Can you work these out from the model? Positions are in its coordinate system, mm. Face numbers are marked on the shaded views. A direction names the side the tool comes from. Give positions to 0.01 mm unless a question says otherwise; leave off trailing zeros. Write each loop counter-clockwise with the first axis right and the second up, starting at its lowest first coordinate (ties: lowest second). Pieces come first, ordered by that corner, then holes.
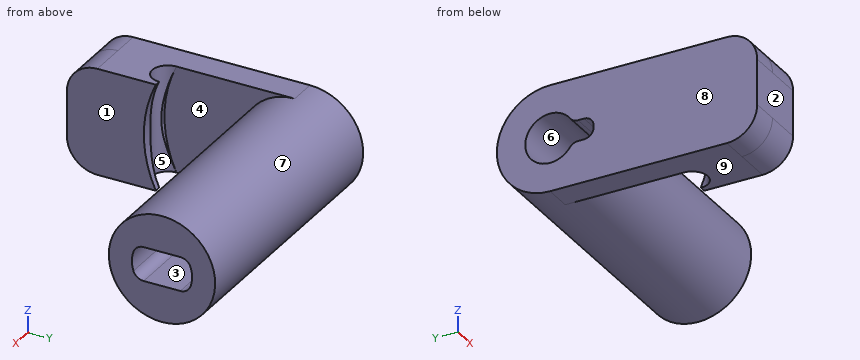
from build123d import *

# Parameters (mm, degrees)
SKETCH1_R           = 8.7376
BOSS_EXTRUDE1_DEPTH = 43.815
BOSS_EXTRUDE3_DEPTH = 4.516000112
FILLET2_R           = 5
BOSS_EXTRUDE4_START = 6.096
BOSS_EXTRUDE4_DEPTH = 6.096
CUT_EXTRUDE8_DEPTH  = 6.096
CUT_EXTRUDE10_DEPTH = 12.192
FILLET11_R          = 1.778
SKETCH25_R          = 2.5527
CUT_EXTRUDE14_DEPTH = 59.168600946
CUT_EXTRUDE15_DEPTH = 21.59
FILLET12_R          = 1.5875


with BuildPart() as part:
    # Sketch1 → Boss-Extrude1 (new body)
    with BuildSketch(Plane.YZ):
        with Locations(Location((0, 0, 0), (0, 0, 270))):
            Circle(SKETCH1_R)
    extrude(amount=BOSS_EXTRUDE1_DEPTH)

    # Sketch10 → Boss-Extrude3 (add)
    with BuildSketch(Plane(origin=(0, 0, 0), x_dir=(0, -1, 0), z_dir=(-1, 0, 0))):
        with BuildLine():
            Line((0, 8.7376), (34.036, 8.7376))
            Line((34.036, 8.7376), (34.036, -8.7376))
            Line((34.036, -8.7376), (0, -8.7376))
            ThreePointArc((0, -8.7376), (8.7376, 0), (0, 8.7376))
        make_face()
    extrude(amount=-BOSS_EXTRUDE3_DEPTH)

    # Fillet2
    fillet2_edges = [part.edges().sort_by_distance(p)[0] for p in [
        (2.258000056, -34.036, 8.7376),
        (2.258000056, -34.036, -8.7376),
    ]]
    fillet(fillet2_edges, radius=FILLET2_R)

    # Sketch15 → Boss-Extrude4 (add)
    with BuildSketch(Plane.YZ.offset(4.516000112).offset(BOSS_EXTRUDE4_START)):
        with BuildLine():
            Line((-18.796, 8.7376), (-29.036, 8.7376))
            ThreePointArc((-29.036, 8.7376), (-32.571533906, 7.273133906), (-34.036, 3.7376))
            Line((-34.036, 3.7376), (-34.036, -3.7376))
            ThreePointArc((-34.036, -3.7376), (-32.571533906, -7.273133906), (-29.036, -8.7376))
            Line((-29.036, -8.7376), (-18.796, -8.7376))
            Line((-18.796, -8.7376), (-18.796, 8.7376))
        make_face()
    extrude(amount=-BOSS_EXTRUDE4_DEPTH)

    # Sketch21 → Cut-Extrude8 (cut)
    with BuildSketch(Plane.YZ.offset(10.612000112)):
        with BuildLine():
            Line((-19.431, -8.7376), (-18.796, -8.7376))
            Line((-18.796, -8.7376), (-18.796, 8.7376))
            Line((-18.796, 8.7376), (-19.431, 8.7376))
            ThreePointArc((-19.431, 8.7376), (-21.405517007, 0), (-19.431, -8.7376))
        make_face()
    extrude(amount=-CUT_EXTRUDE8_DEPTH, mode=Mode.SUBTRACT)

    # Sketch22 → Cut-Extrude10 (cut)
    with BuildSketch(Plane.YZ.offset(43.815)):
        with BuildLine():
            Line((-4.089715516, -2.794), (4.089715516, -2.794))
            ThreePointArc((4.089715516, -2.794), (4.953, 0), (4.089715516, 2.794))
            Line((4.089715516, 2.794), (-4.089715516, 2.794))
            ThreePointArc((-4.089715516, 2.794), (-4.953, 0), (-4.089715516, -2.794))
        make_face()
    extrude(amount=-CUT_EXTRUDE10_DEPTH, mode=Mode.SUBTRACT)

    # Fillet11
    fillet11_edges = [part.edges().sort_by_distance(p)[0] for p in [
        (37.719, 4.089715516, 2.794),
        (37.719, 4.089715516, -2.794),
        (37.719, -4.089715516, -2.794),
        (37.719, -4.089715516, 2.794),
    ]]
    fillet(fillet11_edges, radius=FILLET11_R)

    # Sketch25 → Cut-Extrude14 (cut, through all)
    with BuildSketch(Plane(origin=(0, 0, -8.7376), x_dir=(1, 0, 0), z_dir=(0, 0, -1))):
        with Locations((7.068700112, 19.431)):
            Circle(SKETCH25_R)
    extrude(amount=-CUT_EXTRUDE14_DEPTH, mode=Mode.SUBTRACT)

    # Sketch26 → Cut-Extrude15 (cut)
    with BuildSketch(Plane(origin=(0, 0, 0), x_dir=(0, -1, 0), z_dir=(-1, 0, 0))):
        with BuildLine():
            Line((3.684641875, 1.7145), (7.177141875, 1.7145))
            Line((7.177141875, 1.7145), (7.177141875, -1.7145))
            Line((7.177141875, -1.7145), (3.684641875, -1.7145))
            ThreePointArc((3.684641875, -1.7145), (-4.064, 0), (3.684641875, 1.7145))
        make_face()
    extrude(amount=-CUT_EXTRUDE15_DEPTH, mode=Mode.SUBTRACT)

    # Fillet12
    fillet12_edges = [part.edges().sort_by_distance(p)[0] for p in [
        (10.795, -3.684641875, -1.7145),
        (10.795, -3.684641875, 1.7145),
        (10.795, -7.177141875, 1.7145),
        (10.795, -7.177141875, -1.7145),
    ]]
    fillet(fillet12_edges, radius=FILLET12_R)


solid = part.part
(1) Imagine slicing it at B-B, the plane z = -7.5. Write out the boundary of the cut face in (x, y) (3 decimals).
Returned:
outline: (0, -32.329) - (10.612, -32.329) - (10.612, -19.971) - (9.564, -19.971) arc R2.553 cw to (4.574, -19.971) - (4.516, -19.971) - (4.516, -4.483) - (43.815, -4.483) - (43.815, 4.483) - (0, 4.483) - close
(2) Will these pins go through, and if not, where does the flat tip stop? P1, Ø6, axis at x = 25.5, z = 3.5, coming from the -Y side; P2, Ø4.5, axis at y = -0.5, z = -1, coming from the +X side (3 decimals); P3, Ø6, axis at y = -18, z = 0.5, coming from the +X side; P4, Ø6, axis at y = -24.5, z = 0.5, coming from the +X side.
Returned:
P1: stops at y = -8.72
P2: stops at x = 43.815
P3: stops at x = 4.52
P4: stops at x = 10.61
(3) Imagine slicing it at D-D, the plane y = 2. Write out the boundary of the cut face in (x, z) (3 decimals), plus the area to 3 significant figures.
Returned:
outline: (0, -8.506) - (43.815, -8.506) - (43.815, -2.794) - (31.623, -2.794) - (31.623, 2.794) - (43.815, 2.794) - (43.815, 8.506) - (0, 8.506) - (0, 3.538) - (21.59, 3.538) - (21.59, -3.538) - (0, -3.538) - close
area: 524 mm2
(4) Imagine slicing it at C-C, the plane x = 35. Write out the boundary of the cut face in (y, z).
Returned:
outline: circle Ø17.48 at (0, 0); hole (-4.69, -1.58) arc R1.78 ccw to (-3.01, -2.79) - (3.01, -2.79) arc R1.78 ccw to (4.69, -1.58) arc R4.95 ccw to (4.69, 1.58) arc R1.78 ccw to (3.01, 2.79) - (-3.01, 2.79) arc R1.78 ccw to (-4.69, 1.58) arc R4.95 ccw to start
(5) For the marked faces 5, 6, 7, 8 and 9, which set-ups out of +Z, -Z, +X, -X, +Y, -Y let a thin tool reach every point of the face, with its end or its side?
Returned:
face 5: +Z, -Z
face 6: -X
face 7: +X
face 8: +Z, -Z, -X, +Y, -Y
face 9: -Z, +X, -X, +Y, -Y
(6) If we mould it in two halves opening along Y, with no side actions, what happens to the marked faces 1, 2, 3 and 4? For each: +Y half, -Y half, draft (parallel to the pull), parting line (faces both ways), or undercut.
Returned:
face 1: draft
face 2: -Y half
face 3: undercut
face 4: undercut
(7) If I drill on L1, parallel to Y at x = 7, z = 0; L2, parallel to Y at x = 12.5, z = 0; L3, parallel to X at y = -31, z = -5.25, over which ranges is the centre line in solid material (lowest first)?
Returned:
L1: y = -34.04 to -21.98, -8.74 to -7.18, 4.06 to 8.74
L2: y = -8.74 to -7.18, 4.06 to 8.74
L3: x = 0 to 10.61
